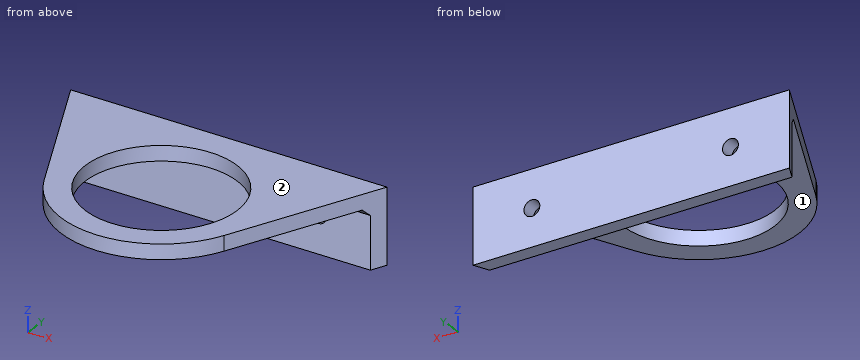
from build123d import *

# Parameters (mm, degrees)
SKETCH_1_R          = 15.15
EXTRUDE_1_DEPTH     = 15
SKETCH_2_W          = 12
SKETCH_2_H          = 38
CUT_EXTRUDE_1_DEPTH = 35
CUT_EXTRUDE_2_REACH = 56.047
SKETCH_3_R          = 1.6
CHAMFER_1_SIZE      = 1.5


with BuildPart() as part:
    # ｽｹｯﾁ1 → ﾎﾞｽ - 押し出し1 (new body)
    with BuildSketch(Plane.XY):
        with BuildLine():
            Line((-18.126155741, -8.452365235), (-31.860019201, 21))
            Line((-31.860019201, 21), (31.860019201, 21))
            Line((31.860019201, 21), (18.126155741, -8.452365235))
            ThreePointArc((18.126155741, -8.452365235), (0, -20), (-18.126155741, -8.452365235))
        make_face()
        Circle(SKETCH_1_R, mode=Mode.SUBTRACT)
    extrude(amount=EXTRUDE_1_DEPTH)

    # ｽｹｯﾁ2 → ｶｯﾄ - 押し出し1 (cut, symmetric)
    with BuildSketch(Plane(origin=(0, 0, 0), x_dir=(0, 0, -1), z_dir=(1, 0, 0))):
        with Locations((-6, -1)):
            Rectangle(SKETCH_2_W, SKETCH_2_H)
    extrude(amount=CUT_EXTRUDE_1_DEPTH, both=True, mode=Mode.SUBTRACT)

    # ｽｹｯﾁ3 → ｶｯﾄ - 押し出し2 (cut, up to next)
    with BuildSketch(Plane(origin=(0, 21, 0), x_dir=(1, 0, 0), z_dir=(0, 1, 0)), mode=Mode.PRIVATE) as cut_extrude_2_sk1:
        with Locations(Location((-20, -7.5, 0), (0, 0, 270))):
            Circle(SKETCH_3_R)
    cut_extrude_2_tool1 = extrude(cut_extrude_2_sk1.sketch, amount=-CUT_EXTRUDE_2_REACH, mode=Mode.PRIVATE) & part.part
    # ｽｹｯﾁ3 → ｶｯﾄ - 押し出し2 (cut, up to next)
    with BuildSketch(Plane(origin=(0, 21, 0), x_dir=(1, 0, 0), z_dir=(0, 1, 0)), mode=Mode.PRIVATE) as cut_extrude_2_sk2:
        with Locations(Location((20, -7.5, 0), (0, 0, 270))):
            Circle(SKETCH_3_R)
    cut_extrude_2_tool2 = extrude(cut_extrude_2_sk2.sketch, amount=-CUT_EXTRUDE_2_REACH, mode=Mode.PRIVATE) & part.part
    add(cut_extrude_2_tool1.solids().sort_by_distance((-20, 21, 7.5))[0], mode=Mode.SUBTRACT)
    add(cut_extrude_2_tool2.solids().sort_by_distance((20, 21, 7.5))[0], mode=Mode.SUBTRACT)

    # 面取り1
    chamfer_1_edges = [part.edges().sort_by_distance(p)[0] for p in [
        (0, 18, 12),
    ]]
    chamfer(chamfer_1_edges, length=CHAMFER_1_SIZE)


solid = part.part
Work out the finished part from the listing and answer in its coordinate system (mm). Face numbers are marked on the shaded views. A direction names the side the tool comes from. Give positions to 0.01 mm unless a question says otherwise; leave off trailing zeros. Loops run counter-clockwise (first coordinate to the right, second up) from the corner with the lowest first, then second, coordinate; pieces in that order, holes last. Notation, with made-up numbers: (-33, -39) -> (22, -39) arc R25 cw to (22, -19) -> close; hole circle Ø8 at (-20, 56.5). An arc over 180 degrees is marked (long way). Use a Markdown table: item, result. Add a question column.
1. Section A-A on z = 7.5 is taken. Determine the outline of the cut face in (x, y).
2. Flat-ended cylindrical pins translate along their axes: pin 1 Ø6 at (y, z) = (12.5, 8.5) entering from +X; pin 2 Ø10 at (x, y) = (11, 2.5) entering from -Z; pin 3 Ø1 at (x, z) = (-1, 9.5) entering from -Y; pin 4 Ø1.5 at (x, z) = (-16.5, 10) entering from -Y. Find the tip coordinate at first contact, or state that the pin passes through.
3. Section D-D on z = 14 is taken. Determine the outline of the cut face in (x, y).
4. Section B-B on x = 0 is taken. Determine the outline of the cut face in (y, z), and give its area (3 significant figures).
5. Section C-C on y = 0 is taken. Determine the outline of the cut face in (x, z).
6. For the marked faces 1 and 2, determine the directions among +Z, -Z, +X, -X, +Y, -Y from which every point of the face is accessible in a straight line to the end or side of a thin tool.
7. Find the intervals of material crossed by probe 1 along Y at (x, z) = (0, 14.1); probe 2 along X at (y, z) = (19.9, 7.5); probe 3 along Z at (x, y) = (11, -14), in increasing order.
Results below:
| question | item | result |
|---|---|---|
| 1 | outline | (-31.86, 21) -> (-30.46, 18) -> (-21.6, 18) -> (-21.6, 21) -> close; (-18.4, 18) -> (18.4, 18) -> (18.4, 21) -> (-18.4, 21) -> close; (21.6, 18) -> (30.46, 18) -> (31.86, 21) -> (21.6, 21) -> close |
| 2 | pin 1 | passes through |
| 2 | pin 2 | stops at z = 12 |
| 2 | pin 3 | stops at y = 18 |
| 2 | pin 4 | stops at y = 17.75 |
| 3 | outline | (-31.86, 21) -> (-18.13, -8.45) arc R20 ccw to (18.13, -8.45) -> (31.86, 21) -> close; hole circle Ø30.3 at (0, 0) |
| 4 | outline | (-20, 12) -> (-15.15, 12) -> (-15.15, 15) -> (-20, 15) -> close; (15.15, 12) -> (16.5, 12) -> (18, 10.5) -> (18, 0) -> (21, 0) -> (21, 15) -> (15.15, 15) -> close |
| 4 | area | 69.2 mm^2 |
| 5 | outline | (-22.07, 12) -> (-15.15, 12) -> (-15.15, 15) -> (-22.07, 15) -> close; (15.15, 12) -> (22.07, 12) -> (22.07, 15) -> (15.15, 15) -> close |
| 6 | face 1 | -Z, +X, -X, -Y |
| 6 | face 2 | +Z, +X, -X, +Y, -Y |
| 7 | probe 1 | y = -20 to -15.15, 15.15 to 21 |
| 7 | probe 2 | x = -31.35 to -21.6, -18.4 to 18.4, 21.6 to 31.35 |
| 7 | probe 3 | z = 12 to 15 |
